from build123d import *

# Parameters (mm, degrees)
BOSS_EXTRUDE1_DEPTH = 25.654
FILLET1_R           = 25.4
FILLET2_R           = 2.54


with BuildPart() as part:
    # Sketch1 → Boss-Extrude1 (new body)
    with BuildSketch(Plane(origin=(0, 0, 0), x_dir=(0, 0, -1), z_dir=(1, 0, 0))):
        Polygon((-6.572, -12.7), (-4.572, -12.7), (-4.572, 0), (4.572, 0), (4.572, -25.4), (6.572, -25.4), (6.572, 3.175), (-6.572, 3.175), align=None)
    extrude(amount=BOSS_EXTRUDE1_DEPTH)

    # Fillet1
    # the kernel refuses this fillet: 25.4 mm, written as the material it takes off along each edge
    with BuildSketch(Plane(origin=(-24.69817807, -12.7, 6.572), x_dir=(0, 0, -1), z_dir=(1, 0, 0))) as fillet1_piece_1:
        with BuildLine():
            CenterArc((25.4, 9.879271228), FILLET1_R, 180, 22.889037196)
            Line((0, 9.879271228), (-0.508, 9.879271228))
            Line((-0.508, 9.879271228), (-0.508, 0))
            Line((-0.508, 0), (0, -0.508))
            ThreePointArc((0, -0.508), (1, -0.508), (1.532, -0.197585425))
            Line((1.532, -0.197585425), (2, 0))
        make_face()
    extrude(amount=75.050356141, mode=Mode.SUBTRACT)
    with BuildSketch(Plane(origin=(-24.69817807, -25.4, -6.572), x_dir=(0, 0, 1), z_dir=(1, 0, 0))) as fillet1_piece_2:
        with BuildLine():
            CenterArc((25.4, -9.879271228), FILLET1_R, 157.110962804, 22.889037196)
            Line((0, -9.879271228), (-0.508, -9.879271228))
            Line((-0.508, -9.879271228), (-0.508, 0))
            Line((-0.508, 0), (0, 0.508))
            ThreePointArc((0, 0.508), (1, 0.508), (1.532, 0.197585425))
            Line((1.532, 0.197585425), (2, 0))
        make_face()
    extrude(amount=75.050356141, mode=Mode.SUBTRACT)

    # Fillet2
    fillet2_edges = [part.edges().sort_by_distance(p)[0] for p in [
        (12.827, 3.175, 6.572),
        (12.827, 3.175, -6.572),
    ]]
    fillet(fillet2_edges, radius=FILLET2_R)


solid = part.part
Design review of the part built by this model. Coordinates are the model's own, in mm. A direction names the side the tool comes from. Coordinates: 2 decimals unless noted, no trailing zeros. Loops run counter-clockwise (first coordinate to the right, second up) from the corner with the lowest first, then second, coordinate; pieces in that order, holes last. Notation, with made-up numbers: (-2, 66) -> (12, 66) arc R24 ccw to (12, 95) -> close; hole circle Ø5 at (76.25, 17). An arc over 180 degrees is marked (long way). Use a Markdown table: item, result. Add a question column.
Item 1: Machinability: for faces 1 (the flat face through (0, -5, -5)), 2 (the flat face through (13, -6, 4.572)), which of the approach directions +Z, -Z, +X, -X, +Y, -Y give a long, thin tool a straight path to every point of the face, cutting with its end or side? Answer none if there is none.
Item 2: The part is to be moulded in two halves that separate along Z. For faces 3 (the flat face through (13, -13, -4.572)), 4 (the flat face through (25.654, -5, -5)), 5 (the cylindrical face through (13.01, 2.41, 5.85)), say which applies: +Z half, -Z half, draft (parallel to the pull), parting line (faces both ways), or undercut.
Item 3: We need section D-D, the plane y = -12. Write out the cut boundary in (x, z).
Item 4: Wall thickness on L1, parallel to Z at x = 12.25, y = -2.5; L2, parallel to Y at x = 12.25, z = 4 (3 decimals); L3, parallel to Z at x = 16, y = -8: over which ranges is each line inside the solid? List them lowest first. Write a range as from..to.
Item 5: We need section A-A, the plane y = -2. Write out the cut boundary in (x, z).
Item 6: Clearance check with flat-ended pins moving along their axes: P1, Ø2, axis at x = 13.5, y = -20.5, coming from the +Z side; P2, Ø1.5, axis at x = 8, y = -18.5, coming from the -Z side; P3, Ø7.5, axis at x = 17, y = -10, coming from the +Z side; P4, Ø5, axis at y = -3, z = 0, coming from the +X side. State where each tip first meets the part, or that it passes through.
Item 7: We need section C-C, the plane z = 0.5. Write out the cut boundary in (x, y) (3 decimals), and give its area (3 significant figures).
Item 8: We need section B-B, the plane x = 3.5. Write out the cut boundary in (y, z) (3 decimals).
Numbers:
| question | item | result |
|---|---|---|
| 1 | face 1 | +Z, -Z, -X, +Y, -Y |
| 1 | face 2 | +X, -X, -Y |
| 2 | face 3 | undercut |
| 2 | face 4 | draft |
| 2 | face 5 | +Z half |
| 3 | outline | (0, -6.57) -> (25.65, -6.57) -> (25.65, -4.57) -> (0, -4.57) -> close; (0, 4.57) -> (25.65, 4.57) -> (25.65, 4.86) -> (0, 4.86) -> close |
| 4 | L1 | z = -6.57..-4.57, 4.57..6.57 |
| 4 | L2 | y = 0..3.175 |
| 4 | L3 | z = -6.57..-4.57, 4.57..6.04 |
| 5 | outline | (0, -6.57) -> (25.65, -6.57) -> (25.65, -4.57) -> (0, -4.57) -> close; (0, 4.57) -> (25.65, 4.57) -> (25.65, 6.57) -> (0, 6.57) -> close |
| 6 | P1 | stops at z = -4.57 |
| 6 | P2 | stops at z = -6.47 |
| 6 | P3 | stops at z = 6.34 |
| 6 | P4 | passes through |
| 7 | outline | (0, 0) -> (25.654, 0) -> (25.654, 3.175) -> (0, 3.175) -> close |
| 7 | area | 81.5 mm^2 |
| 8 | outline | (-25.4, -4.572) arc R25.4 ccw to (-15.521, -6.572) -> (0.635, -6.572) arc R2.54 ccw to (3.175, -4.032) -> (3.175, 4.032) arc R2.54 ccw to (0.635, 6.572) -> (-2.821, 6.572) arc R25.4 ccw to (-12.7, 4.572) -> (0, 4.572) -> (0, -4.572) -> close |
